Can you work these out from the drawing? Everything is in mm from the part's minimum corner. A direction names the side the tool comes from. Coordinates: 2 decimals unless noted, no trailing zeros. Loops run counter-clockwise (first coordinate to the right, second up) from the corner with the lowest first, then second, coordinate; pieces in that order, holes last. Notation, with made-up numbers: (56.25, 15.5) - (98.25, 15.5) arc R26 cw to (98.25, 46.5) - close; hole circle Ø8 at (41.25, 80). An arc over 180 degrees is marked (long way). Use CSV: the item, a comma, the result in double quotes.
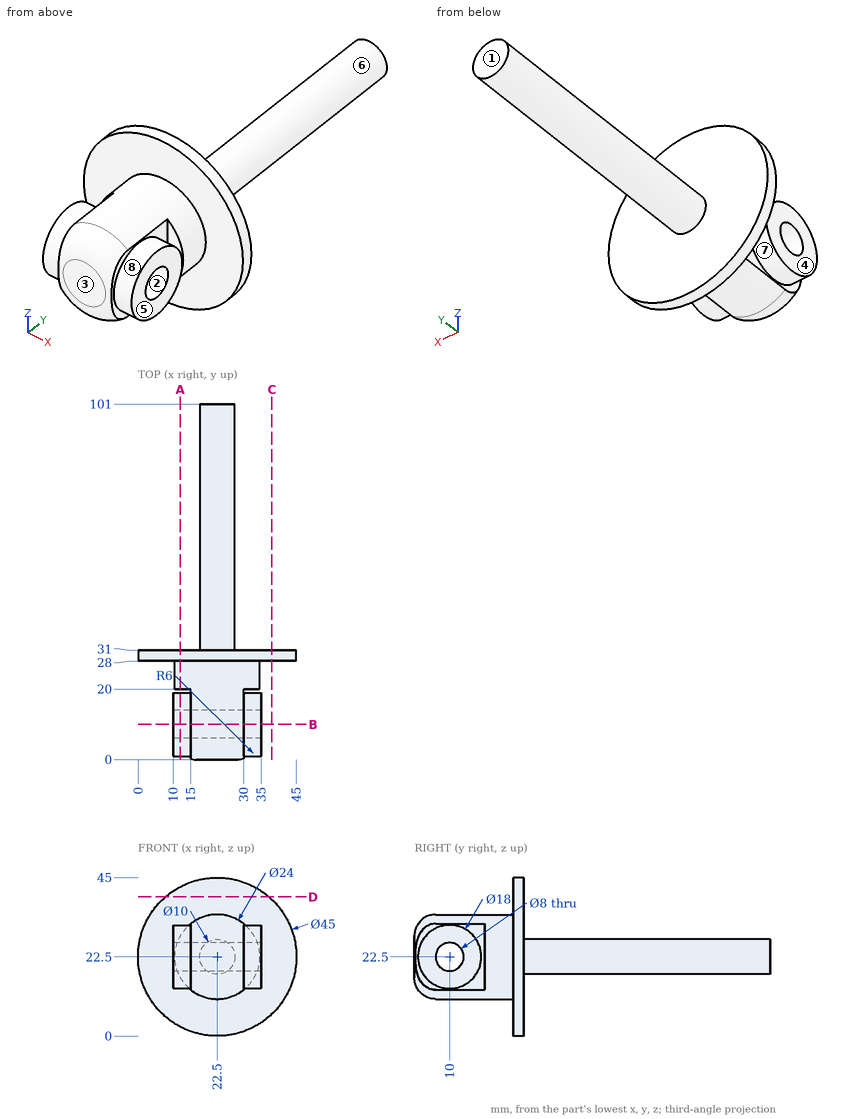
(1) Suppose I cut it at D-D (z = 39.5). Write out the boundary of the cut face in (x, y).
Computed:
outline,"(7.76, 28) - (37.24, 28) - (37.24, 31) - (7.76, 31) - close"
(2) Will these pins go through, and if not, where does the flat tip stop? pin 1 (14.5 mm diameter, centred on y = 6.5, z = 23, fed in from +X); pin 2 (1.5 mm diameter, centred on x = 27, y = 53, fed in from -Z); pin 3 (6 mm diameter, centred on x = 33, z = 5.5, fed in from -Y); pin 4 (10 mm diameter, centred on y = 59.5, z = 34.5, fed in from +X).
Computed:
pin 1,"stops at x = 35"
pin 2,"stops at z = 19.19"
pin 3,"stops at y = 28"
pin 4,"passes through"
(3) Please list where these lines run through material, in increasing order: line 1 (Y direction, x = 17, z = 22.5); line 2 (Y direction, x = 5, z = 35.5); line 3 (Y direction, x = 13, z = 26).
Computed:
line 1,"y = 0 to 6, 14 to 31"
line 2,"y = 28 to 31"
line 3,"y = 1.71 to 8.06, 11.94 to 18.29, 20 to 31"
(4) Suppose I cut it at B-B (y = 10). Write out the boundary of the cut face in (x, z).
Computed:
outline,"(10, 13.5) - (15, 13.5) - (15, 13.13) arc R12 ccw to (30, 13.13) - (30, 13.5) - (35, 13.5) - (35, 18.5) - (10, 18.5) - close; (10, 26.5) - (35, 26.5) - (35, 31.5) - (30, 31.5) - (30, 31.87) arc R12 ccw to (15, 31.87) - (15, 31.5) - (10, 31.5) - close"
(5) Suppose I cut it at A-A (x = 12). Write out the boundary of the cut face in (y, z).
Computed:
outline,"circle Ø18 at (10, 22.5); (20, 16.69) - (28, 16.69) - (28, 2.6) - (31, 2.6) - (31, 42.4) - (28, 42.4) - (28, 28.31) - (20, 28.31) - close; hole circle Ø8 at (10, 22.5)"
(6) Which directions (+Z, -Z, +X, -X, +Y, -Y) give clear straight access to the entire face, cutting with the end or side of a thin tool? Please do the marked faces 4, 5, 6, 7 and 8.
Computed:
face 4,"+Z, -Z, -X, -Y"
face 5,"+Z, -Z, +X, -Y"
face 6,"+Y"
face 7,"-X"
face 8,"+X"
(7) Suppose I cut it at C-C (x = 38). Write out the boundary of the cut face in (y, z), plus the area to 3 significant figures.
Computed:
outline,"(28, 6.19) - (31, 6.19) - (31, 38.81) - (28, 38.81) - close"
area,"97.9 mm²"
(8) Thinking about a two-plate mould opening in Y: for the marked faces 1, 2 and 3, which applies, +Y half, -Y half, draft (parallel to the pull), parting line (faces both ways), or undercut?
Computed:
face 1,"+Y half"
face 2,"undercut"
face 3,"-Y half"
